from build123d import *

# Parameters (mm, degrees)
SKETCH1_R           = 4.5
SKETCH1_R_2         = 2
BOSS_EXTRUDE1_DEPTH = 2
CUT_EXTRUDE1_START  = 2
SKETCH2_R           = 4
SKETCH2_R_2         = 2.5
CUT_EXTRUDE1_DEPTH  = 0.2
CUT_EXTRUDE3_START  = -2
SKETCH2_2_R         = 4
SKETCH2_2_R_2       = 2.5
CUT_EXTRUDE3_DEPTH  = 0.2
CHAMFER1_SIZE       = 0.05


with BuildPart() as part:
    # Sketch1 → Boss-Extrude1 (new body, symmetric)
    with BuildSketch(Plane(origin=(0, 0, 0), x_dir=(1, 0, 0), z_dir=(0, 1, 0))):
        Circle(SKETCH1_R)
        Circle(SKETCH1_R_2, mode=Mode.SUBTRACT)
    extrude(amount=BOSS_EXTRUDE1_DEPTH, both=True)

    # Sketch2 → Cut-Extrude1 (cut)
    with BuildSketch(Plane(origin=(0, 0, 0), x_dir=(1, 0, 0), z_dir=(0, 1, 0)).offset(CUT_EXTRUDE1_START)):
        Circle(SKETCH2_R)
        Circle(SKETCH2_R_2, mode=Mode.SUBTRACT)
    extrude(amount=-CUT_EXTRUDE1_DEPTH, mode=Mode.SUBTRACT)

    # Sketch2<2> → Cut-Extrude3 (cut)
    with BuildSketch(Plane(origin=(0, 0, 0), x_dir=(1, 0, 0), z_dir=(0, 1, 0)).offset(CUT_EXTRUDE3_START)):
        Circle(SKETCH2_2_R)
        Circle(SKETCH2_2_R_2, mode=Mode.SUBTRACT)
    extrude(amount=CUT_EXTRUDE3_DEPTH, mode=Mode.SUBTRACT)

    # Chamfer1
    chamfer1_edges = [part.edges().sort_by_distance(p)[0] for p in [
        (-4, 2, 0),
        (-2.5, 2, 0),
        (-2.5, -2, 0),
        (-4, -2, 0),
        (-4.5, -2, 0),
        (-4.5, 2, 0),
        (-2, -2, 0),
        (-2, 2, 0),
    ]]
    chamfer(chamfer1_edges, length=CHAMFER1_SIZE)


solid = part.part
Design review of the part built by this model. Coordinates are the model's own, in mm. A direction names the side the tool comes from. Coordinates: 2 decimals unless noted, no trailing zeros. Order: outer loops, then holes, each group sorted by start corner. A loop starts at its lowest first (then second) coordinate and runs counter-clockwise, first axis right, second up. Notation, with made-up numbers: (-15, 76) -> (17, 76) arc R28 ccw to (17, 96) -> close; hole circle Ø9 at (15.25, -39.5). An arc over 180 degrees is marked (long way). One line per item, written item: value.
1) We need section A-A, the plane y = -0.7. Give the boundary of the cut face in (x, z), then the cut area to 3 significant figures.
Output values:
outline: circle Ø9 at (0, 0); hole circle Ø4 at (0, 0)
area: 51.1 mm2
2) Clearance check with flat-ended pins moving along their axes: P1, Ø1, axis at y = -1, z = -1, coming from the +X side; P2, Ø2, axis at x = -2, y = -1.5, coming from the +Z side. State where each tip first meets the part, or that it passes through.
Output values:
P1: stops at x = 4.47
P2: stops at z = 4.39
3) To check wall thickness, follow probe 1 along X at (y, z) = (-1.85, 0); probe 2 along X at (y, z) = (-1.75, 0). State the ranges of each line that lie inside material, in increasing order. Write a range as [from, to].
Output values:
probe 1: x = [-4.5, -4], [-2.5, -2], [2, 2.5], [4, 4.5]
probe 2: x = [-4.5, -2], [2, 4.5]
4) Draft analysis for pull direction Z (two halves, no side actions). For faces 3 (the face through (-0.59, 0.03, -4.46)), 4 (the face through (2, 1.8, -2)), 5 (the face through (-1, 2, 2)), state which applies: +Z half, -Z half, draft (parallel to the pull), parting line (faces both ways), or undercut.
Output values:
face 3: parting line
face 4: undercut
face 5: draft
5) Machinability: for faces 1 (the face through (2, -1.8, -2)), 2 (the face through (-1, -2, 2)), which of the approach directions +Z, -Z, +X, -X, +Y, -Y give a long, thin tool a straight path to every point of the face, cutting with its end or side? Answer none if there is none.
Output values:
face 1: -Y
face 2: +Z, -Z, +X, -X, -Y
